Could you check a few things on this drawing? It's one solid part, dimensions in mm from its lowest x, y, z. Give positions to 0.01 mm unless a question says otherwise; leave off trailing zeros. Write each loop counter-clockwise with the first axis right and the second up, starting at its lowest first coordinate (ties: lowest second). Pieces come first, ordered by that corner, then holes. Notation, with made-up numbers: M 85.5,38.25 L 91.5,38.25 A20 ccw 91.5,61.25 Z; hole C 2,19 d6. An arc over 180 degrees is marked long. Answer as CSV lines item,"result". Start each with the question number.
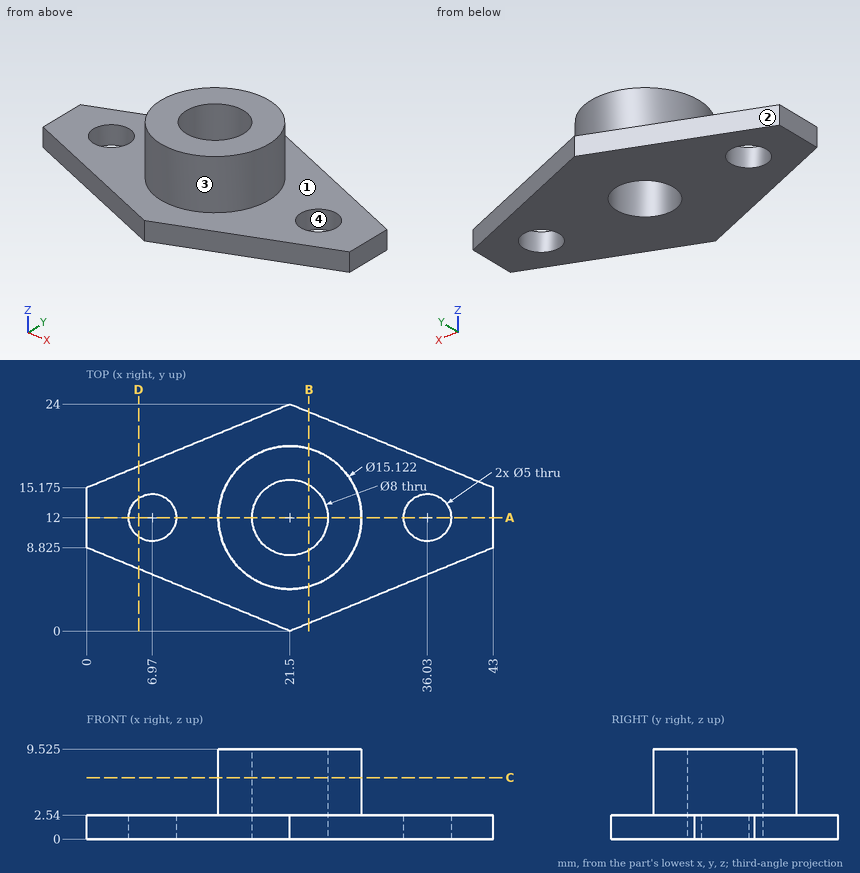
1) I want a section at C-C, the plane z = 6.5. Please give me the cut outline in (x, y).
2) I want a section at B-B, the plane x = 23.5. Please give me the cut outline in (y, z) (1 decimal).
3) Thinking about a two-plate mould opening in Y: for the marked faces 1, 2, 3 and 4, which applies, released by +Y, released by -Y, zero draft, split by the parting line, or undercut?
4) I need wall thicknesses on L1, parallel to Y at x = 21.5, z = 7.75; L2, parallel to X at y = 11.75, z = 9; L3, parallel to X at y = 10.75, z = 0.5 (1 decimal). Which ranges of each line are inside material? Lowest first, please. Write a range as from..to.
5) I'm going to push flat-ended pins straight in: P1, Ø1, axis at y = 17, z = 7, coming from the -X side (1 decimal); P2, Ø4, axis at x = 13, z = 5.5, coming from the +Y side; P3, Ø6.5, axis at x = 6.97, y = 12, coming from the +Z side. Where does each tip first touch, or does it pass through?
6) I want a section at A-A, the plane y = 12. Please give me the cut outline in (x, z) (1 decimal), then the cut area to 3 significant figures.
7) I want a section at D-D, the plane x = 5.5. Please give me the cut outline in (y, z).
Values found:
1,outline,"C 21.5,12 d15.12; hole C 21.5,12 d8"
2,outline,"M 0.8,0 L 8.5,0 L 8.5,9.5 L 4.7,9.5 L 4.7,2.5 L 0.8,2.5 Z; M 15.5,0 L 23.2,0 L 23.2,2.5 L 19.3,2.5 L 19.3,9.5 L 15.5,9.5 Z"
3,face 1,"zero draft"
3,face 2,"released by +Y"
3,face 3,"split by the parting line"
3,face 4,"undercut"
4,L1,"y = 4.44..8, 16..19.56"
4,L2,"x = 13.94..17.51, 25.49..29.06"
4,L3,"x = 0..4.8, 9.1..17.7, 25.3..33.9, 38.2..43"
5,P1,"stops at x = 15.4"
5,P2,"stops at y = 15.86"
5,P3,"stops at z = 2.54"
6,outline,"M 0,0 L 4.5,0 L 4.5,2.5 L 0,2.5 Z; M 9.5,0 L 17.5,0 L 17.5,9.5 L 13.9,9.5 L 13.9,2.5 L 9.5,2.5 Z; M 25.5,0 L 33.5,0 L 33.5,2.5 L 29.1,2.5 L 29.1,9.5 L 25.5,9.5 Z; M 38.5,0 L 43,0 L 43,2.5 L 38.5,2.5 Z"
6,area,"113 mm²"
7,outline,"M 6.57,0 L 9.98,0 L 9.98,2.54 L 6.57,2.54 Z; M 14.02,0 L 17.43,0 L 17.43,2.54 L 14.02,2.54 Z"
